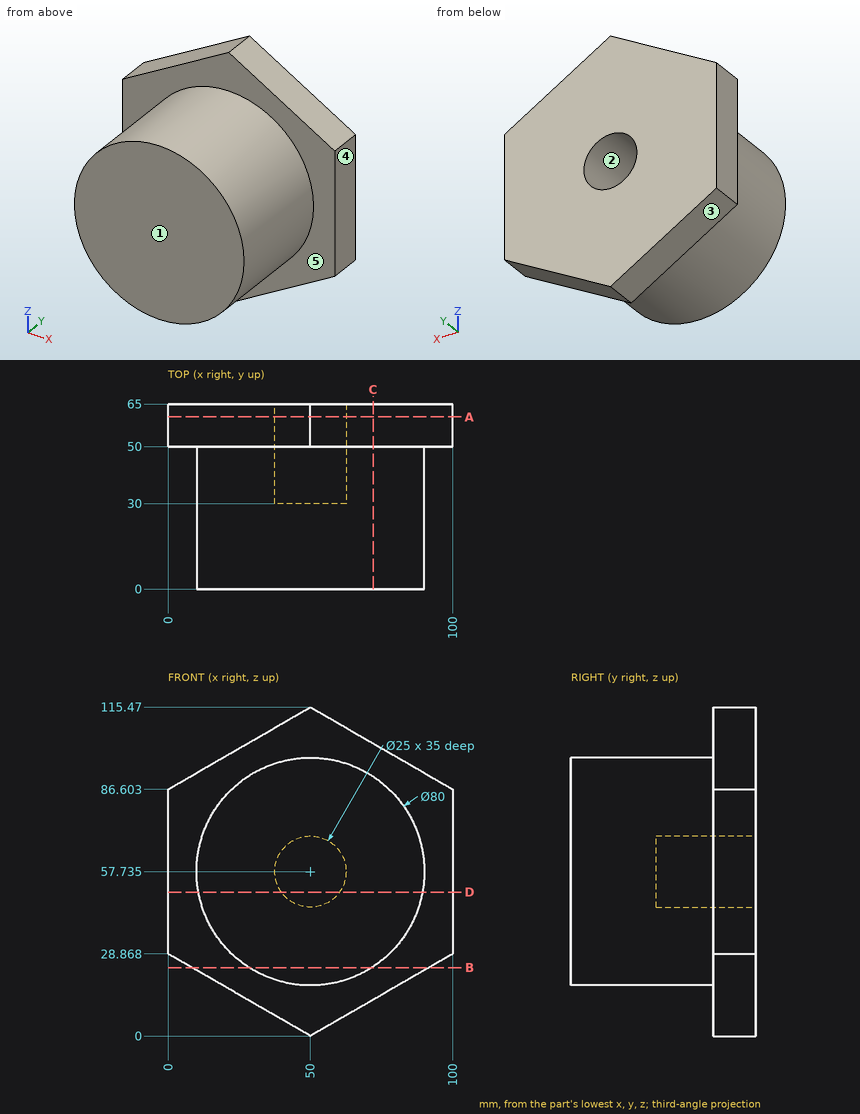
Geometry: see drawing. Coordinates: mm, zero at the bounding-box minimum. A direction names the side the tool comes from. Round coordinates to 2 decimals unless told otherwise and drop trailing zeros. Loops run counter-clockwise (first coordinate to the right, second up) from the corner with the lowest first, then second, coordinate; pieces in that order, holes last. Notation, with made-up numbers: M 79,61 L 108,61 A27 ccw 108,98 Z; hole C 68.25,-6.5 d7. An arc over 180 degrees is marked long. Use a Markdown table: item, result. Add a question column.
1. Line query: line 1 (Z direction, x = 50, y = 49) (1 decimal); line 2 (Y direction, x = 63.5, z = 106.5); line 3 (Y direction, x = 59, z = 52.5). Output: solid intervals per line, ascending.
2. Mould query, pull axis Z, two halves, no side actions, for the marked faces 1, 2 and 3. Classes: pulls with the +Z half, pulls with the -Z half, needs draft (parallel to the pull), parting line crosses it, or undercut.
3. Section query C-C on x = 72. Return the cut outline in (y, z).
4. Contact query for flat-ended pins moving along their axis: P1, Ø3, axis at y = 31.5, z = 59.5, coming from the +X side; P2, Ø1.5, axis at y = 19, z = 44, coming from the -X side; P3, Ø2, axis at x = 81, z = 92, coming from the -Y side; P4, Ø5, axis at y = 8, z = 13, coming from the -X side. Output: stop coordinate, or through.
5. Section query B-B on z = 24. Return the cut outline in (x, y), then the cut area to 3 significant figures.
6. Section query D-D on z = 50.5. Return the cut outline in (x, y).
7. Reachability of the marked faces 4 and 5 from +Z, -Z, +X, -X, +Y, -Y: full face, straight path, thin tool, end or side. Return the list, or none.
8. Section query A-A on y = 60.5. Return the cut outline in (x, z) (1 decimal).
Reported:
| question | item | result |
|---|---|---|
| 1 | line 1 | z = 17.7 to 45.2, 70.2 to 97.7 |
| 1 | line 2 | y = 50 to 65 |
| 1 | line 3 | y = 0 to 30 |
| 2 | face 1 | needs draft |
| 2 | face 2 | undercut |
| 2 | face 3 | pulls with the -Z half |
| 3 | outline | M 0,24.33 L 50,24.33 L 50,12.7 L 65,12.7 L 65,102.77 L 50,102.77 L 50,91.14 L 0,91.14 Z |
| 4 | P1 | stops at x = 90 |
| 4 | P2 | stops at x = 12.17 |
| 4 | P3 | stops at y = 50 |
| 4 | P4 | passes through |
| 5 | outline | M 8.43,50 L 28.51,50 L 28.51,0 L 71.49,0 L 71.49,50 L 91.57,50 L 91.57,65 L 8.43,65 Z |
| 5 | area | 3,400 mm² |
| 6 | outline | M 0,50 L 10.66,50 L 10.66,0 L 89.34,0 L 89.34,50 L 100,50 L 100,65 L 60.19,65 L 60.19,30 L 39.81,30 L 39.81,65 L 0,65 Z |
| 7 | face 4 | +Z, -Z, +X, +Y, -Y |
| 7 | face 5 | -Y |
| 8 | outline | M 0,28.9 L 50,0 L 100,28.9 L 100,86.6 L 50,115.5 L 0,86.6 Z; hole C 50,57.7 d25 |
